Input: part model. Units: mm. Frame: model coordinates. A direction names the side the tool comes from. Round coordinates to 2 decimals unless told otherwise and drop trailing zeros. Loops run counter-clockwise (first coordinate to the right, second up) from the corner with the lowest first, then second, coordinate; pieces in that order, holes last.
1) Section C-C, the plane x = 28.5. Return loops of the section in (y, z).
2) Draft query along Y for faces 1 (the face through (-58.23, 49.52, 3.94)), 2 (the face through (50.84, 54.02, 3.94)), 3 (the face through (-58.28, -49.4, 3.94)), 4 (the face through (-54.16, 54.02, 3.94)). Return one class per face: pulls with the +Y half, pulls with the -Y half, needs draft (parallel to the pull), parting line crosses it, or undercut.
3) Section D-D, the plane z = 26. Return loops of the section in (x, y).
4) Section A-A, the plane x = 52.5. Return loops of the section in (y, z).
5) Section B-B, the plane z = 3.5. State how many separate pieces and enclosed holes the cut face has, and give its area (3 significant figures).
6) Access query for faces 5 (the face through (46.646, 50.221, 3.944)), 6 (the face through (1, 49, 15)), 7 (the face through (57.5, 46.07, 14.79)), 8 (the face through (46.571, -50.157, 3.944)). Directions: +Z, -Z, +X, -X, +Y, -Y. A direction counts if a zero-diameter tool reaches every point of the face in a straight line with its end or side. Return the directions, or none.
7) Ray query, line 1 along Y through (x, z) = (-52.5, 4.25); line 2 along Y through (x, z) = (-26, 25); line 3 along X through (y, z) = (-15.5, 8). Return the intervals inside material, ascending.
8) First-contact query: pin 1 (15 mm diameter, centred on x = 12, z = 14.5, fed in from -Y); pin 2 (6 mm diameter, centred on x = -52.5, y = 52.5, fed in from +Z); pin 3 (2 mm diameter, centred on x = -15.5, z = 19.5, fed in from +Y). Flat tips, straight axial feed; report the tip coordinate or a pass-through.
from build123d import *

# Parameters (mm, degrees)
F1_DEPTH = 30
F0_R     = 2.25
F2_DEPTH = 8
F3_R     = 800
F4_DEPTH = 121.001


with BuildPart() as f1:
    # F0 (on Top) → F1 (new body)
    with BuildSketch(Plane.XY):
        with BuildLine():
            ThreePointArc((60.0523881171, -44.8703582176), (60.3871168285, -43.7061254575), (60.5, -42.5))
            Line((60.5, -42.5), (60.5, 42.5))
            ThreePointArc((60.5, 42.5), (60.3871168285, 43.7061254575), (60.0523881171, 44.8703582176))
            ThreePointArc((60.0523881171, 44.8703582176), (57.6635141317, 47.8692331116), (54, 49))
            Line((54, 49), (43.3724318682, 49))
            Line((43.3724318682, 49), (-43.3724318682, 49))
            Line((-43.3724318682, 49), (-54, 49))
            ThreePointArc((-54, 49), (-57.6635141317, 47.8692331116), (-60.0523881171, 44.8703582176))
            ThreePointArc((-60.0523881171, 44.8703582176), (-60.3871168285, 43.7061254575), (-60.5, 42.5))
            Line((-60.5, 42.5), (-60.5, -42.5))
            ThreePointArc((-60.5, -42.5), (-60.3871168285, -43.7061254575), (-60.0523881171, -44.8703582176))
            ThreePointArc((-60.0523881171, -44.8703582176), (-57.6635141317, -47.8692331116), (-54, -49))
            Line((-54, -49), (-43.3724318682, -49))
            Line((-43.3724318682, -49), (43.3724318682, -49))
            Line((43.3724318682, -49), (54, -49))
            ThreePointArc((54, -49), (57.6635141317, -47.8692331116), (60.0523881171, -44.8703582176))
        make_face()
        with BuildLine():
            Line((-54, 47.5), (54, 47.5))
            ThreePointArc((54, 47.5), (57.5355339059, 46.0355339059), (59, 42.5))
            Line((59, 42.5), (59, -42.5))
            ThreePointArc((59, -42.5), (57.5355339059, -46.0355339059), (54, -47.5))
            Line((54, -47.5), (-54, -47.5))
            ThreePointArc((-54, -47.5), (-57.5355339059, -46.0355339059), (-59, -42.5))
            Line((-59, -42.5), (-59, 42.5))
            ThreePointArc((-59, 42.5), (-57.5355339059, 46.0355339059), (-54, 47.5))
        make_face(mode=Mode.SUBTRACT)
    extrude(amount=F1_DEPTH)

    # F0 (on Top) → F2 (join)
    with BuildSketch(Plane.XY):
        with BuildLine():
            Line((-54, 49), (-43.3724318682, 49))
            ThreePointArc((-43.3724318682, 49), (-46.6086291695, 50.1885662767), (-48.30625248, 53.1891891892))
            ThreePointArc((-48.30625248, 53.1891891892), (-52.0537295479, 56.7265047833), (-56.457330692, 54.0498496038))
            Line((-56.457330692, 54.0498496038), (-60.0523881171, 44.8703582176))
            ThreePointArc((-60.0523881171, 44.8703582176), (-57.6635141317, 47.8692331116), (-54, 49))
        make_face()
        with Locations((-52.5, 52.5)):
            Circle(F0_R, mode=Mode.SUBTRACT)
        with BuildLine():
            ThreePointArc((-48.30625248, -53.1891891892), (-46.6086291695, -50.1885662767), (-43.3724318682, -49))
            Line((-43.3724318682, -49), (-54, -49))
            ThreePointArc((-54, -49), (-57.6635141317, -47.8692331116), (-60.0523881171, -44.8703582176))
            Line((-60.0523881171, -44.8703582176), (-56.457330692, -54.0498496038))
            ThreePointArc((-56.457330692, -54.0498496038), (-52.0537295479, -56.7265047833), (-48.30625248, -53.1891891892))
        make_face()
        with Locations((-52.5, -52.5)):
            Circle(F0_R, mode=Mode.SUBTRACT)
        with BuildLine():
            Line((56.457330692, -54.0498496038), (60.0523881171, -44.8703582176))
            ThreePointArc((60.0523881171, -44.8703582176), (57.6635141317, -47.8692331116), (54, -49))
            Line((54, -49), (43.3724318682, -49))
            ThreePointArc((43.3724318682, -49), (46.6086291695, -50.1885662767), (48.30625248, -53.1891891892))
            ThreePointArc((48.30625248, -53.1891891892), (52.0537295479, -56.7265047833), (56.457330692, -54.0498496038))
        make_face()
        with Locations((52.5, -52.5)):
            Circle(F0_R, mode=Mode.SUBTRACT)
        with BuildLine():
            ThreePointArc((54, 49), (57.6635141317, 47.8692331116), (60.0523881171, 44.8703582176))
            Line((60.0523881171, 44.8703582176), (56.457330692, 54.0498496038))
            ThreePointArc((56.457330692, 54.0498496038), (52.0537295479, 56.7265047833), (48.30625248, 53.1891891892))
            ThreePointArc((48.30625248, 53.1891891892), (46.6086291695, 50.1885662767), (43.3724318682, 49))
            Line((43.3724318682, 49), (54, 49))
        make_face()
        with Locations((52.5, 52.5)):
            Circle(F0_R, mode=Mode.SUBTRACT)
    extrude(amount=F2_DEPTH)

    # F3 (on face) → F4 (cut, through all)
    with BuildSketch(Plane(origin=(-60.5, 0, 0), x_dir=(0, -1, 0), z_dir=(-1, 0, 0))):
        with Locations((0, 828.5885987165)):
            Circle(F3_R)
    extrude(amount=-F4_DEPTH, mode=Mode.SUBTRACT)


solid = f1.part
Final values:
1. outline: (-49, 0) - (-47.5, 0) - (-47.5, 30) - (-49, 30) - close; (47.5, 0) - (49, 0) - (49, 30) - (47.5, 30) - close
2. face 1: pulls with the +Y half
2. face 2: undercut
2. face 3: pulls with the -Y half
2. face 4: undercut
3. outline: (-60.5, -42.5) arc R6.5 ccw to (-54, -49) - (54, -49) arc R6.5 ccw to (60.5, -42.5) - (60.5, 42.5) arc R6.5 ccw to (54, 49) - (-54, 49) arc R6.5 ccw to (-60.5, 42.5) - close; hole (-59, -42.5) arc R5 ccw to (-54, -47.5) - (54, -47.5) arc R5 ccw to (59, -42.5) - (59, 42.5) arc R5 ccw to (54, 47.5) - (-54, 47.5) arc R5 ccw to (-59, 42.5) - close
4. outline: (-56.75, 0) - (-54.75, 0) - (-54.75, 8) - (-56.75, 8) - close; (-50.25, 0) - (-47.5, 0) - (-47.5, 30) - (-49, 30) - (-49, 8) - (-50.25, 8) - close; (47.5, 0) - (50.25, 0) - (50.25, 8) - (49, 8) - (49, 30) - (47.5, 30) - close; (54.75, 0) - (56.75, 0) - (56.75, 8) - (54.75, 8) - close
5. separate pieces: 1
5. enclosed holes: 5
5. area: 850 mm2
6. face 5: +Z, -Z, +Y
6. face 6: +Z, +Y
6. face 7: +Z, -Z
6. face 8: +Z, -Z, -Y
7. line 1: y = -56.75 to -54.75, -50.25 to -47.5, 47.5 to 50.25, 54.75 to 56.75
7. line 2: y = -49 to -47.5, 47.5 to 49
7. line 3: x = -60.5 to -59, 59 to 60.5
8. pin 1: stops at y = -49
8. pin 2: stops at z = 8
8. pin 3: stops at y = 49
